from build123d import *

# Parameters (mm, degrees)
SKETCH_1_R          = 1.5
SKETCH_1_R_2        = 0.75
EXTRUDE_1_DEPTH     = 2.3
SKETCH_2_R          = 4.35
SKETCH_2_R_2        = 2.45
EXTRUDE_2_DEPTH     = 3.2
CUT_EXTRUDE_START   = -1.2
SKETCH_3_R          = 4.4
SKETCH_3_R_2        = 3.425
SKETCH_3_R_3        = 2.725
SKETCH_3_R_4        = 1.5
CUT_EXTRUDE_1_DEPTH = 1.2


with BuildPart() as part:
    # Sketch 1 → Бобышка-Вытянуть1 (new body)
    with BuildSketch(Plane(origin=(0, 0, 0), x_dir=(1, 0, 0), z_dir=(0, 1, 0))):
        with BuildLine():
            Line((4.438538611, 4), (16.5, 2.5))
            ThreePointArc((16.5, 2.5), (19, 0), (16.5, -2.5))
            Line((16.5, -2.5), (4.438538611, -4))
            ThreePointArc((4.438538611, -4), (0, -5.975), (-4.438538611, -4))
            Line((-4.438538611, -4), (-16.5, -2.5))
            ThreePointArc((-16.5, -2.5), (-19, 0), (-16.5, 2.5))
            Line((-16.5, 2.5), (-4.438538611, 4))
            ThreePointArc((-4.438538611, 4), (0, 5.975), (4.438538611, 4))
        make_face()
        with Locations(Location((0, 0, 0), (0, 0, 270))):
            Circle(SKETCH_1_R, mode=Mode.SUBTRACT)
        with Locations(Location((10.3, 0, 0), (0, 0, 270))):
            Circle(SKETCH_1_R_2, mode=Mode.SUBTRACT)
        with Locations(Location((13.35, 0, 0), (0, 0, 270))):
            Circle(SKETCH_1_R_2, mode=Mode.SUBTRACT)
        with Locations(Location((16.4, 0, 0), (0, 0, 270))):
            Circle(SKETCH_1_R_2, mode=Mode.SUBTRACT)
        with Locations(Location((-10.3, 0, 0), (0, 0, 270))):
            Circle(SKETCH_1_R_2, mode=Mode.SUBTRACT)
        with Locations(Location((-13.35, 0, 0), (0, 0, 270))):
            Circle(SKETCH_1_R_2, mode=Mode.SUBTRACT)
        with Locations(Location((-16.4, 0, 0), (0, 0, 270))):
            Circle(SKETCH_1_R_2, mode=Mode.SUBTRACT)
        with Locations(Location((7.25, 0, 0), (0, 0, 270))):
            Circle(SKETCH_1_R_2, mode=Mode.SUBTRACT)
        with Locations(Location((-7.25, 0, 0), (0, 0, 270))):
            Circle(SKETCH_1_R_2, mode=Mode.SUBTRACT)
    extrude(amount=EXTRUDE_1_DEPTH)

    # Эскиз2 → Бобышка-Вытянуть2 (add)
    with BuildSketch(Plane.XZ):
        with Locations(Location((0, 0, 0), (0, 0, 90))):
            Circle(SKETCH_2_R)
        with Locations(Location((0, 0, 0), (0, 0, 270))):
            Circle(SKETCH_2_R_2, mode=Mode.SUBTRACT)
    extrude(amount=EXTRUDE_2_DEPTH)

    # Эскиз3 → Вырез-Вытянуть1 (cut)
    # profile 1 of 2: a face of its own
    with BuildSketch(Plane(origin=(0, 2.3, 0), x_dir=(1, 0, 0), z_dir=(0, 1, 0)).offset(CUT_EXTRUDE_START)):
        with Locations(Location((0, 0, 0), (0, 0, 270))):
            Circle(SKETCH_3_R)
        with Locations(Location((0, 0, 0), (0, 0, 270))):
            Circle(SKETCH_3_R_2, mode=Mode.SUBTRACT)
    # profile 2 of 2: a face of its own
    with BuildSketch(Plane(origin=(0, 2.3, 0), x_dir=(1, 0, 0), z_dir=(0, 1, 0)).offset(CUT_EXTRUDE_START)):
        with Locations(Location((0, 0, 0), (0, 0, 270))):
            Circle(SKETCH_3_R_3)
        with Locations(Location((0, 0, 0), (0, 0, 270))):
            Circle(SKETCH_3_R_4, mode=Mode.SUBTRACT)
    extrude(amount=CUT_EXTRUDE_1_DEPTH, mode=Mode.SUBTRACT)


solid = part.part
Design review of the part built by this model. Coordinates are the model's own, in mm. A direction names the side the tool comes from. Coordinates: 2 decimals unless noted, no trailing zeros. Order: outer loops, then holes, each group sorted by start corner. A loop starts at its lowest first (then second) coordinate and runs counter-clockwise, first axis right, second up. Notation, with made-up numbers: (21, 33) -> (57, 33) arc R34 ccw to (57, 63) -> close; hole circle Ø2 at (55.25, -19.5). An arc over 180 degrees is marked (long way). Use one line per item in the form item = value. Start each with the question number.
(1) For probe 1 along X at (y, z) = (2, -1); probe 2 along Y at (x, z) = (-9.5, 0.75); probe 3 along X at (y, z) = (-0.65, -1.5), list the stretches that pass through material, from the lowest coordinate up.
(2) The part is to be moulded in two halves that separate along X. For faces 4 (the cylindrical face through (19, 1, 0)), 5 (the cylindrical face through (0.45, 0.54, 1.43)), 6 (the cylindrical face through (0.07, 1.134, 5.975)), say which applies: +X half, -X half, draft (parallel to the pull), parting line (faces both ways), or undercut.
(3) Add section A-A on x = 7.25. State the section outline as (y, z) points, plus the area to 3 significant figures.
(4) Add section D-D on x = 13.35. State the section outline as (y, z) points, plus the area to 3 significant figures.
(5) Insertion check: pin 1 (2 mm diameter, centred on x = 7.25, z = 0, fed in from -Y); pin 2 (1.5 mm diameter, centred on y = -1.5, z = 3.5, fed in from +X). Each pin has a flat end and moves straight along its axis. Give the tip position at first contact, or say it passes through.
(6) For faces 1 (the cylindrical face through (2.65, -1.58, -3.45)), 2 (the cylindrical face through (4.363, 1.692, -0.573)), 3 (the cylindrical face through (-12.718, 1.134, 0.403)), list the 3-axis set-ups (+Z, -Z, +X, -X, +Y, -Y) from which the entire face can be reached by the end or side of a thin tool; tool diameter is ignored.
(7) Add section C-C on z = -0.25. Give the number of separate pieces and of enclosed holes in the cut face, plus the area to 3 significant figures.
(8) Add section B-B on y = -1.45. State the section outline as (x, z) points, plus the area to 3 significant figures.
Answer block:
q1.probe_1 = -18.79 to -4.28, -3.28 to -2.53, 2.53 to 3.28, 4.28 to 18.79
q1.probe_2 = 0 to 2.3
q1.probe_3 = -4.08 to -1.94, 1.94 to 4.08
q2.face_4 = +X half
q2.face_5 = undercut
q2.face_6 = parting line
q3.outline = (0, -3.65) -> (2.3, -3.65) -> (2.3, -0.75) -> (0, -0.75) -> close; (0, 0.75) -> (2.3, 0.75) -> (2.3, 3.65) -> (0, 3.65) -> close
q3.area = 13.3 mm²
q4.outline = (0, -2.89) -> (2.3, -2.89) -> (2.3, -0.75) -> (0, -0.75) -> close; (0, 0.75) -> (2.3, 0.75) -> (2.3, 2.89) -> (0, 2.89) -> close
q4.area = 9.85 mm²
q5.pin_1 = 0
q5.pin_2 = 3.37
q6.face_1 = -Y
q6.face_2 = +Y
q6.face_3 = +Y, -Y
q7.separate_pieces = 10
q7.enclosed_holes = 0
q7.area = 61.4 mm²
q8.outline = circle Ø8.7 at (0, 0); hole circle Ø4.9 at (0, 0)
q8.area = 40.6 mm²
